Source: three-view drawing plus pictorial views. Frame: mm from the lowest corner of the part. A direction names the side the tool comes from. Give positions to 0.01 mm unless a question says otherwise; leave off trailing zeros. Loops run counter-clockwise (first coordinate to the right, second up) from the corner with the lowest first, then second, coordinate; pieces in that order, holes last. Notation, with made-up numbers: M -19.5,-16.75 L 25.5,-16.75 A21 cw 25.5,-6.75 Z; hole C 88,86 d10. An arc over 180 degrees is marked long. Write item = value, one per line.
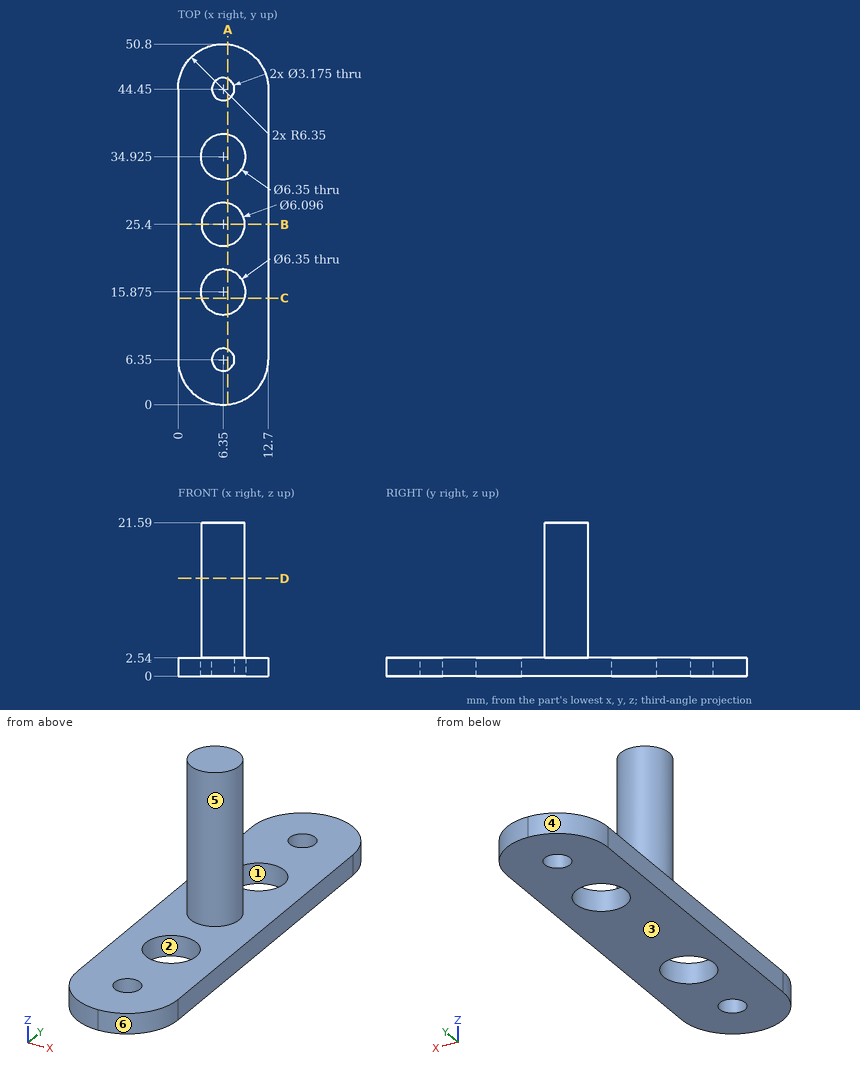
1. Material intervals for probe 1 along Y at (x, z) = (6.35, 0.8); probe 2 along Y at (x, z) = (6.5, 8.25); probe 3 along X at (y, z) = (25.5, 7.25), sorted ascending. Write a range as from..to.
Derived:
probe_1 = 0..4.76, 7.94..12.7, 19.05..31.75, 38.1..42.86, 46.04..50.8
probe_2 = 22.36..28.44
probe_3 = 3.3..9.4
2. Reachability of the marked faces 5 and 6 from +Z, -Z, +X, -X, +Y, -Y: full face, straight path, thin tool, end or side. Return the list, or none.
Derived:
face_5 = +Z
face_6 = +Z, -Z, +X, -Y
3. Cut plane C-C, the plane y = 15. Return the cut outline in (x, z), then the cut area to 3 significant figures.
Derived:
outline = M 0,0 L 3.3,0 L 3.3,2.54 L 0,2.54 Z; M 9.4,0 L 12.7,0 L 12.7,2.54 L 9.4,2.54 Z
area = 16.8 mm²
4. Cut plane B-B, the plane y = 25.4. Return the cut outline in (x, z).
Derived:
outline = M 0,0 L 12.7,0 L 12.7,2.54 L 9.4,2.54 L 9.4,21.59 L 3.3,21.59 L 3.3,2.54 L 0,2.54 Z
5. First-contact query: pin 1 Ø4 at (y, z) = (23, 16) entering from +X; pin 2 Ø3 at (x, z) = (4.5, 13) entering from -Y; pin 3 Ø7.5 at (x, y) = (6.35, 34.925) entering from +Z. Flat tips, straight axial feed; report the tip coordinate or a pass-through.
Derived:
pin_1 = 9.37
pin_2 = 22.37
pin_3 = 2.54
6. Cut plane A-A, the plane x = 7. Return the cut outline in (y, z), then the cut area to 3 significant figures.
Derived:
outline = M 0.03,0 L 4.9,0 L 4.9,2.54 L 0.03,2.54 Z; M 7.8,0 L 12.77,0 L 12.77,2.54 L 7.8,2.54 Z; M 18.98,0 L 31.82,0 L 31.82,2.54 L 28.38,2.54 L 28.38,21.59 L 22.42,21.59 L 22.42,2.54 L 18.98,2.54 Z; M 38.03,0 L 43,0 L 43,2.54 L 38.03,2.54 Z; M 45.9,0 L 50.77,0 L 50.77,2.54 L 45.9,2.54 Z
area = 196 mm²
7. Cut plane D-D, the plane z = 13.75. Return the cut outline in (x, y), then the cut area to 3 significant figures.
Derived:
outline = C 6.35,25.4 d6.1
area = 29.2 mm²
8. Pull-direction query (X, two-part tool) for the marked faces 1, 2, 3 and 4; classes: +X half, -X half, draft (parallel to the pull), parting line (faces both ways), or undercut.
Derived:
face_1 = undercut
face_2 = undercut
face_3 = draft
face_4 = -X half
